Build history of the part. All positions in model axes, mm. A direction names the side the tool comes from. Round coordinates to 2 decimals unless told otherwise and drop trailing zeros. Loops run counter-clockwise (first coordinate to the right, second up) from the corner with the lowest first, then second, coordinate; pieces in that order, holes last. Notation, with made-up numbers: M -2.5,46.5 L 23.5,46.5 A20 ccw 23.5,81.5 Z; hole C 83,-32.5 d5. An arc over 180 degrees is marked long. One line per item, written item: value.
```python
from build123d import *

# Parameters (mm, degrees)
F1_W         = 36
F1_H         = 36
F2_DEPTH     = 9
F3_T         = -2
F4_START     = 7
F0_W         = 34
F0_H         = 34
F4_DEPTH     = 3
F5_R         = 1
F6_R         = 0.5
F7_T1_DEPTH  = 10.5
F7_S5_W      = 1
F7_S5_H      = 1
F7_T6_DEPTH  = 1
F7_S11_W     = 1
F7_S11_H     = 1
F7_T12_DEPTH = 1
F7_S17_W     = 1
F7_S17_H     = 1
F7_T18_DEPTH = 1
F7_S23_W     = 1
F7_S23_H     = 1
F7_T24_DEPTH = 1
F9_DEPTH     = 2
F11_START    = -1.5
F10_W        = 12.2
F10_H        = 20.1
F11_DEPTH    = 2.5
F13_DEPTH    = 2
F14_R        = 1.5
F15_DEPTH    = 4.001
F16_R        = 0.5
F17_R        = 0.5


# Not quite as in the source:
# - a fillet or chamfer that OpenCascade refuses, or shapes differently, is made with other operations: its cross-section is extruded or revolved along the edge and cut away or added


with BuildPart() as f2:
    # F1 (on Top) → F2 (new body)
    with BuildSketch(Plane.XY):
        Rectangle(F1_W, F1_H)
    extrude(amount=F2_DEPTH)

    # F3
    f3_openings = [f2.faces().sort_by_distance(p)[0] for p in [
        (0, 0, 9),
    ]]
    offset(amount=F3_T, openings=f3_openings)

    # F0 (on Top) → F4 (cut)
    with BuildSketch(Plane.XY.offset(F4_START)):
        Rectangle(F0_W, F0_H)
    extrude(amount=F4_DEPTH, mode=Mode.SUBTRACT)

    # F5
    f5_edges = [f2.edges().sort_by_distance(p)[0] for p in [
        (18, 0, 0),
        (0, 18, 0),
        (-18, 0, 0),
        (0, -18, 0),
    ]]
    fillet(f5_edges, radius=F5_R)

    # F6
    f6_edges = [f2.edges().sort_by_distance(p)[0] for p in [
        (0, 16, 2),
        (-16, 0, 2),
        (0, -16, 2),
        (16, 0, 2),
        (-16, 16, 4.5),
        (16, 16, 4.5),
        (17, 17, 8),
        (17, -17, 8),
        (16, -16, 4.5),
        (-17, -17, 8),
        (-16, -16, 4.5),
        (-17, 17, 8),
    ]]
    fillet(f6_edges, radius=F6_R)

    # F7: fillet of radius 1 on 4 edges, made by hand

    # F7_s2 → F7_t1 (cut)
    with BuildSketch(Plane.XY.offset(1)):
        with BuildLine():
            ThreePointArc((-18, -17), (-17.7071067812, -17.7071067812), (-17, -18))
            Line((-17, -18), (-18, -18))
            Line((-18, -18), (-18, -17))
        make_face()
        with BuildLine():
            ThreePointArc((17, 18), (17.7071067812, 17.7071067812), (18, 17))
            Line((18, 17), (18, 18))
            Line((18, 18), (17, 18))
        make_face()
        with BuildLine():
            ThreePointArc((18, -17), (17.7071067812, -17.7071067812), (17, -18))
            Line((17, -18), (18, -18))
            Line((18, -18), (18, -17))
        make_face()
        with BuildLine():
            ThreePointArc((-17, 18), (-17.7071067812, 17.7071067812), (-18, 17))
            Line((-18, 17), (-18, 18))
            Line((-18, 18), (-17, 18))
        make_face()
    extrude(amount=F7_T1_DEPTH, mode=Mode.SUBTRACT)


with BuildPart() as f7_tool4:
    # F7_s5 → F7_t6 (new body)
    with BuildSketch(Plane.XZ.offset(-17)):
        with Locations((-17.5, 0.5)):
            Rectangle(F7_S5_W, F7_S5_H)
    extrude(amount=-F7_T6_DEPTH)

    # F7_s7 → F7_t8 (revolve, cut)
    with BuildSketch(Plane(origin=(-17, 17, 1), x_dir=(0.7071067812, 0, 0.7071067812), z_dir=(-0.7071067812, 0, 0.7071067812))):
        with BuildLine():
            ThreePointArc((0, -1), (1, 0), (0, 1))
            Line((0, 1), (0, -1))
        make_face()
    revolve(axis=Axis((-17, 17, 1), (0, 1, 0)), mode=Mode.SUBTRACT)


with BuildPart() as f2_1:
    add(f2.part)

    # F7_t3: cut F7_tool4
    add(f7_tool4.part, mode=Mode.SUBTRACT)


with BuildPart() as f7_tool10:
    # F7_s11 → F7_t12 (new body)
    with BuildSketch(Plane.YZ.offset(17)):
        with Locations((-17.5, 0.5)):
            Rectangle(F7_S11_W, F7_S11_H)
    extrude(amount=F7_T12_DEPTH)

    # F7_s13 → F7_t14 (revolve, cut)
    with BuildSketch(Plane(origin=(17, -17, 1), x_dir=(0, 0.7071067812, 0.7071067812), z_dir=(0, 0.7071067812, -0.7071067812))):
        with BuildLine():
            ThreePointArc((0, -1), (1, 0), (0, 1))
            Line((0, 1), (0, -1))
        make_face()
    revolve(axis=Axis((17, -17, 1), (1, 0, 0)), mode=Mode.SUBTRACT)


with BuildPart() as f2_2:
    add(f2_1.part)

    # F7_t9: cut F7_tool10
    add(f7_tool10.part, mode=Mode.SUBTRACT)


with BuildPart() as f7_tool16:
    # F7_s17 → F7_t18 (new body)
    with BuildSketch(Plane.XZ.offset(-17)):
        with Locations((17.5, 0.5)):
            Rectangle(F7_S17_W, F7_S17_H)
    extrude(amount=-F7_T18_DEPTH)

    # F7_s19 → F7_t20 (revolve, cut)
    with BuildSketch(Plane(origin=(17, 17, 1), x_dir=(-0.7071067812, 0, 0.7071067812), z_dir=(-0.7071067812, 0, -0.7071067812))):
        with BuildLine():
            ThreePointArc((0, -1), (1, 0), (0, 1))
            Line((0, 1), (0, -1))
        make_face()
    revolve(axis=Axis((17, 17, 1), (0, 1, 0)), mode=Mode.SUBTRACT)


with BuildPart() as f2_3:
    add(f2_2.part)

    # F7_t15: cut F7_tool16
    add(f7_tool16.part, mode=Mode.SUBTRACT)


with BuildPart() as f7_tool22:
    # F7_s23 → F7_t24 (new body)
    with BuildSketch(Plane.YZ.offset(-17)):
        with Locations((-17.5, 0.5)):
            Rectangle(F7_S23_W, F7_S23_H)
    extrude(amount=-F7_T24_DEPTH)

    # F7_s25 → F7_t26 (revolve, cut)
    with BuildSketch(Plane(origin=(-17, -17, 1), x_dir=(0, 0.7071067812, 0.7071067812), z_dir=(0, -0.7071067812, 0.7071067812))):
        with BuildLine():
            ThreePointArc((0, -1), (1, 0), (0, 1))
            Line((0, 1), (0, -1))
        make_face()
    revolve(axis=Axis((-17, -17, 1), (-1, 0, 0)), mode=Mode.SUBTRACT)


with BuildPart() as f2_4:
    add(f2_3.part)

    # F7_t21: cut F7_tool22
    add(f7_tool22.part, mode=Mode.SUBTRACT)

    # F8 (on Top) → F9 (join)
    with BuildSketch(Plane.XY):
        with BuildLine():
            ThreePointArc((-11, -11), (-10.4142135624, -12.4142135624), (-9, -13))
            Line((-9, -13), (9, -13))
            ThreePointArc((9, -13), (10.4142135624, -12.4142135624), (11, -11))
            Line((11, -11), (11, 7))
            ThreePointArc((11, 7), (9.5355339059, 10.5355339059), (6, 12))
            Line((6, 12), (-6, 12))
            ThreePointArc((-6, 12), (-9.5355339059, 10.5355339059), (-11, 7))
            Line((-11, 7), (-11, -11))
        make_face()
    extrude(amount=-F9_DEPTH)

    # F10 (on Top) → F11 (cut)
    with BuildSketch(Plane.XY.offset(F11_START)):
        with Locations((0, -2.95)):
            Rectangle(F10_W, F10_H)
    extrude(amount=-F11_DEPTH, mode=Mode.SUBTRACT)

    # F12 (on face) → F13 (cut)
    with BuildSketch(Plane.XY.offset(2)):
        Polygon((-0.3596221451, 3.0790699753), (-2.8463638912, 1.2280930742), (-2.4867417461, -1.850976901), (0.3596221451, -3.0790699753), (2.8463638912, -1.2280930742), (2.4867417461, 1.850976901), align=None)
    extrude(amount=-F13_DEPTH, mode=Mode.SUBTRACT)

    # F14 (on face) → F15 (cut, through all)
    with BuildSketch(Plane.XY.offset(2)):
        Circle(F14_R)
    extrude(amount=-F15_DEPTH, mode=Mode.SUBTRACT)

    # F16
    f16_edges = [f2_4.edges().sort_by_distance(p)[0] for p in [
        (11, -2, 0),
        (6.1, 7.1, -1.75),
        (-6.1, 7.1, -1.75),
    ]]
    fillet(f16_edges, radius=F16_R)

    # F17
    f17_edges = [f2_4.edges().sort_by_distance(p)[0] for p in [
        (7.55, -13, -2),
    ]]
    fillet(f17_edges, radius=F17_R)


solid = f2_4.part
```
Item 1: Slice it at B-B, the plane y = -5.5. Give the cut face in (x, z).
Check values:
outline: M -18,1 A1 ccw -17,0 L -11.5,0 A0.5 cw -11,-0.5 L -11,-1.5 A0.5 ccw -10.5,-2 L -6.1,-2 L -6.1,-1.5 L 6.1,-1.5 L 6.1,-2 L 10.5,-2 A0.5 ccw 11,-1.5 L 11,-0.5 A0.5 cw 11.5,0 L 17,0 A1 ccw 18,1 L 18,9 L 17,9 L 17,7 L 16,7 L 16,2.5 A0.5 cw 15.5,2 L -15.5,2 A0.5 cw -16,2.5 L -16,7 L -17,7 L -17,9 L -18,9 Z
Item 2: Pull direction X, two halves, no side cores. Call faces 4 (the face through (1.2, 1.4, 0)), 5 (the face through (-10.43, -12.4, -0.99)), 6 (the face through (17.699, 17.715, 4.944)): pulls with the +X half, pulls with the -X half, needs draft (parallel to the pull), parting line crosses it, or undercut.
Check values:
face 4: undercut
face 5: pulls with the -X half
face 6: pulls with the +X half
Item 3: Drop flat-ended pins along their axis: P1, Ø1.1, axis at y = -1, z = -1, coming from the -X side; P2, Ø3.5, axis at x = 0, y = 0, coming from the -Z side; P3, Ø0.8, axis at x = 2, z = -1, coming from the +Y side. Give the stop position or say it passes through.
Check values:
P1: stops at x = -11
P2: stops at z = -1.5
P3: stops at y = 12
Item 4: Wall check: line 1 along Y through (x, z) = (0, -0.75); line 2 along Y through (x, z) = (-1, 2.5). Give the ranges that are in metal, low to high.
Check values:
line 1: y = -13 to -1.5, 1.5 to 12
line 2: y = -18 to -16, 16 to 18
Item 5: Slice it at C-C, the plane x = -13. Give the cut face in (y, z), and give its area (3 significant figures).
Check values:
outline: M -18,1 A1 ccw -17,0 L 17,0 A1 ccw 18,1 L 18,9 L 17,9 L 17,7 L 16,7 L 16,2.5 A0.5 cw 15.5,2 L -15.5,2 A0.5 cw -16,2.5 L -16,7 L -17,7 L -17,9 L -18,9 Z
area: 95.7 mm2
Item 6: Which spindle directions (+Z, -Z, +X, -X, +Y, -Y) get a long thin tool onto all of the face, cutting with end or side? Do faces 1 (the face through (0, 12, -1)), 2 (the face through (17, 0, 8)), 3 (the face through (10, 10, -1)). Say none if no direction does.
Check values:
face 1: -Z, +X, -X, +Y
face 2: +Z
face 3: -Z, +X, +Y
Item 7: Slice it at A-A, the plane z = 8.25. Give the cut face in (x, y).
Check values:
outline: M -18,-17 A1 ccw -17,-18 L 17,-18 A1 ccw 18,-17 L 18,17 A1 ccw 17,18 L -17,18 A1 ccw -18,17 Z; hole M -17,-16.5 A0.5 ccw -16.5,-17 L 16.5,-17 A0.5 ccw 17,-16.5 L 17,16.5 A0.5 ccw 16.5,17 L -16.5,17 A0.5 ccw -17,16.5 Z
